from build123d import *

# Parameters (mm, degrees)
F1_DEPTH = 63.5
F0_W     = 49.9602150655
F0_H     = 19.05
F2_DEPTH = 25.4
F3_DEPTH = 7.9375
F4_R     = 5.08


with BuildPart() as f1:
    # F0 (on Front) → F1 (new body, symmetric)
    with BuildSketch(Plane.XZ):
        Polygon((-41.275, -9.525), (41.275, -9.525), (41.275, 9.525), (22.225, 9.525), (-41.275, 9.525), align=None)
    extrude(amount=F1_DEPTH, both=True)

    # F0 (on Front) → F2 (join, symmetric)
    with BuildSketch(Plane.XZ):
        with BuildLine():
            Line((22.225, 9.525), (41.275, 9.525))
            Line((41.275, 9.525), (41.275, 27.0002))
            ThreePointArc((41.275, 27.0002), (45.9246798487, 38.2255201513), (57.15, 42.8752))
            Line((57.15, 42.8752), (60.325, 42.8752))
            Line((60.325, 42.8752), (60.325, 61.9252))
            Line((60.325, 61.9252), (57.15, 61.9252))
            add(Edge.make_bspline(
                [(52.6185648508, 61.6299808322), (54.1767284716, 61.7748193582), (55.6895521193, 61.8740152427), (57.15, 61.9252)],
                knots=[106.7587971819, 106.7587971819, 106.7587971819, 106.7587971819, 111.5045361635, 111.5045361635, 111.5045361635, 111.5045361635], degree=3))
            ThreePointArc((52.6185648508, 61.6299808322), (30.9010381388, 50.0381605479), (22.225, 27.0002))
            Line((22.225, 27.0002), (22.225, 9.525))
        make_face()
        with Locations((85.3051075328, 52.4002)):
            Rectangle(F0_W, F0_H)
        Polygon((110.2852150655, 42.8752), (60.325, 42.8752), (60.325, 34.925), (111.125, 34.925), (111.125, 66.675), (60.325, 66.675), (60.325, 61.9252), (110.2852150655, 61.9252), align=None)
    extrude(amount=F2_DEPTH, both=True)

    # F0 (on Front) → F3 (join, symmetric)
    with BuildSketch(Plane.XZ):
        with BuildLine():
            add(Edge.make_bspline(
                [(-41.275, 9.525), (-40.4300702784, 32.0156986362), (17.5665582788, 58.3717344605), (52.6185648508, 61.6299808322)],
                knots=[0, 0, 0, 0, 106.7587971819, 106.7587971819, 106.7587971819, 106.7587971819], degree=3))
            Line((-41.275, 9.525), (22.225, 9.525))
            Line((22.225, 9.525), (22.225, 27.0002))
            ThreePointArc((22.225, 27.0002), (30.9010381388, 50.0381605479), (52.6185648508, 61.6299808322))
        make_face()
    extrude(amount=F3_DEPTH, both=True)

    # F4
    f4_edges = [f1.edges().sort_by_distance(p)[0] for p in [
        (41.275, -63.5, 0),
        (41.275, 63.5, 0),
        (58.7375, -25.4, 42.8752),
        (-41.275, -63.5, 0),
        (-41.275, 63.5, 0),
        (-41.275, 0, -9.525),
    ]]
    fillet(f4_edges, radius=F4_R)


solid = f1.part
Geometry: final body of the model. Coordinates: model frame, mm. A direction names the side the tool comes from. Give positions to 0.01 mm unless a question says otherwise; leave off trailing zeros. Order: outer loops, then holes, each group sorted by start corner. A loop starts at its lowest first (then second) coordinate and runs counter-clockwise, first axis right, second up. Notation, with made-up numbers: (88, 67.5) - (138, 67.5) arc R35 cw to (138, 102.5) - close; hole circle Ø10 at (60, 61.5). An arc over 180 degrees is marked (long way). Use CSV: the item, a comma, the result in double quotes.
1. Material intervals for line 1 along Z through (x, y) = (13.5, -56) (3 decimals); line 2 along Y through (x, z) = (17.5, 42); line 3 along X through (y, z) = (12, 27) (3 decimals), sorted ascending. Write a range as from..to.
Answers below:
line 1,"-9.525..9.525"
line 2,"-7.94..7.94"
line 3,"22.225..41.275"
2. Contact query for flat-ended pins moving along their axis: pin 1 (8 mm diameter, centred on x = 46.5, z = 20.5, fed in from -Y); pin 2 (1.4 mm diameter, centred on y = 8.5, z = 65.5, fed in from -X) (3 decimals); pin 3 (5 mm diameter, centred on y = -18.5, z = 22.5, fed in from -X) (3 decimals); pin 4 (14.5 mm diameter, centred on y = -9, z = 41, fed in from -X). Output: stop coordinate, or through.
Answers below:
pin 1,"through"
pin 2,"x = 60.325"
pin 3,"x = 22.225"
pin 4,"x = -22.21"
3. Access query for faces 1 (the face through (31.135, -16.791, 50.302)), 2 (the face through (-4, 7.938, 30)), 3 (the face through (58.76, -23.95, 44.4)). Directions: +Z, -Z, +X, -X, +Y, -Y. A direction counts if a zero-diameter tool reaches every point of the face in a straight line with its end or side. Return the directions, or none.
Answers below:
face 1,"+Z, -X, -Y"
face 2,"+Z, -X, +Y"
face 3,"-Z, -Y"
4. Section query B-B (y = 53.5). Output: boundary loops of the cut face in (x, z) (3 decimals), plus the area to 3 significant figures.
Answers below:
outline,"(-41.275, -4.445) arc R5.08 ccw to (-36.195, -9.525) - (41.275, -9.525) - (41.275, 9.525) - (-41.275, 9.525) - close"
area,"1,570 mm2"
5. Section query C-C (x = 98). Output: boundary loops of the cut face in (y, z) (3 decimals), plus the area to 3 significant figures.
Answers below:
outline,"(-25.4, 34.925) - (25.4, 34.925) - (25.4, 66.675) - (-25.4, 66.675) - close"
area,"1,610 mm2"
6. Mould query, pull axis Z, two halves, no side actions, for faces 4 (the face through (60.325, 0, 64)), 5 (the face through (39.75, -23.95, 18.38)), 6 (the face through (31.135, 16.547, 50.302)). Classes: +Z half, -Z half, draft (parallel to the pull), parting line (faces both ways), or undercut.
Answers below:
face 4,"draft"
face 5,"undercut"
face 6,"+Z half"
7. Section query A-A (z = -2). Output: boundary loops of the cut face in (x, y) (3 decimals), plus the area to 3 significant figures.
Answers below:
outline,"(-41.275, -58.42) arc R5.08 ccw to (-36.195, -63.5) - (36.195, -63.5) arc R5.08 ccw to (41.275, -58.42) - (41.275, 58.42) arc R5.08 ccw to (36.195, 63.5) - (-36.195, 63.5) arc R5.08 ccw to (-41.275, 58.42) - close"
area,"10,500 mm2"
